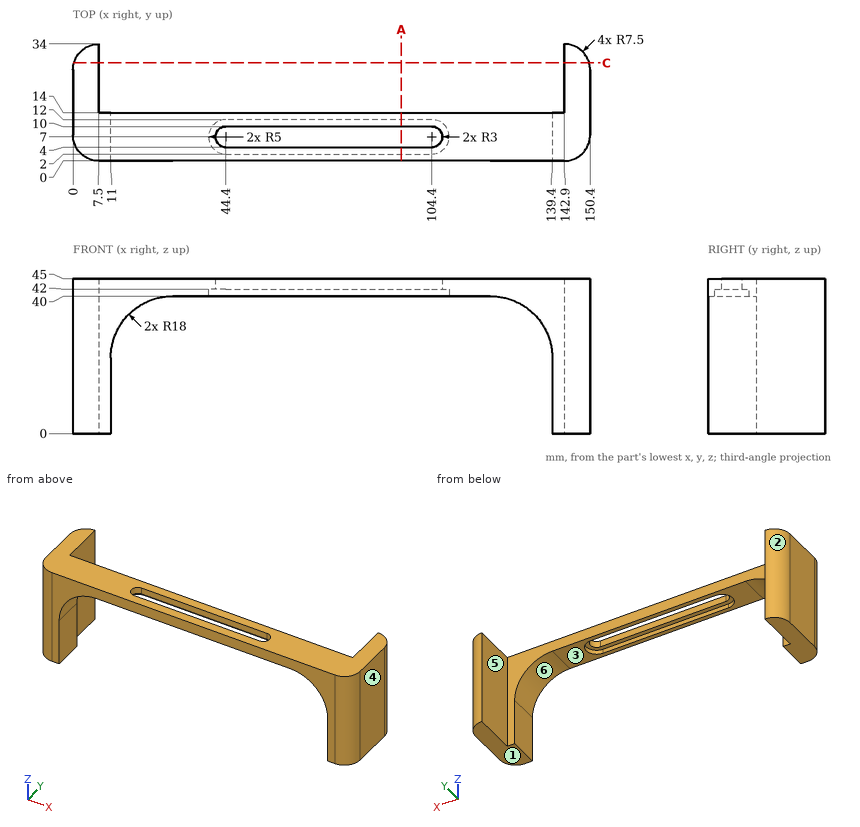
Study the drawing (mm; zero at the part's minimum x, y, z) and answer. A direction names the side the tool comes from. Give positions to 0.01 mm unless a question says otherwise; leave off trailing zeros. Loops run counter-clockwise (first coordinate to the right, second up) from the corner with the lowest first, then second, coordinate; pieces in that order, holes last. Notation, with made-up numbers: (84, 21.25) - (134, 21.25) arc R19 ccw to (134, 42.25) - close; hole circle Ø5 at (-30, 31.5). An arc over 180 degrees is marked (long way). Answer as CSV lines item,"result". Start each with the question number.
1) Which of the six approach directions +Z, -Z, +X, -X, +Y, -Y give full straight-line access (tool end or side, diameter ignored) to the marked faces 4, 5 and 6?
2) Find section A-A (x = 95.5). Write down the section's boundary in (y, z), then the cut area to 3 significant figures.
3) Straight lines are drawn through the part: L1, parallel to X at y = 20, z = 36; L2, parallel to Y at x = 140.5, z = 17; L3, parallel to X at y = 30, z = 13. For each, find the intervals that lie inside material, in ascending order. Write a range as from..to.
4) Determine the mould class of the marked faces 1, 2 and 3 for opening direction X: released by +X, released by -X, zero draft, split by the parting line, or undercut.
5) Each of these flat-tipped pins is pushed along its axis until it touches: pin 1 Ø1.5 at (x, z) = (85.5, 43.5) entering from +Y; pin 2 Ø15.5 at (x, y) = (52, 4.5) entering from -Z. Where does it stop, or does it pass through?
6) Find section C-C (y = 28.5). Write down the section's boundary in (x, z), then the cut area to 3 significant figures.
Findings below:
1,face 4,"+Z, -Z, +X, +Y, -Y"
1,face 5,"+Z, -Z, +Y"
1,face 6,"-Z, +Y, -Y"
2,outline,"(0, 40) - (2, 40) - (2, 42) - (4, 42) - (4, 45) - (0, 45) - close; (10, 42) - (12, 42) - (12, 40) - (14, 40) - (14, 45) - (10, 45) - close"
2,area,"32.0 mm^2"
3,L1,"0..7.5, 142.9..150.4"
3,L2,"0..14"
3,L3,"0.87..7.5, 142.9..149.53"
4,face 1,"zero draft"
4,face 2,"released by -X"
4,face 3,"undercut"
5,pin 1,"y = 14"
5,pin 2,"z = 40"
6,outline,"(0.27, 0) - (7.5, 0) - (7.5, 45) - (0.27, 45) - close; (142.9, 0) - (150.13, 0) - (150.13, 45) - (142.9, 45) - close"
6,area,"651 mm^2"
